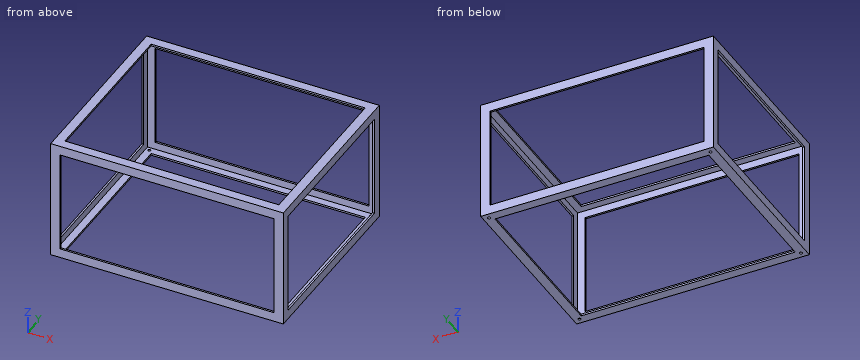
```python
from build123d import *

# Parameters (mm, degrees)
SKETCH1_W           = 250
SKETCH1_H           = 130
BOSS_EXTRUDE1_DEPTH = 200
SKETCH2_W           = 246
SKETCH2_H           = 126
CUT_EXTRUDE1_DEPTH  = 198
SKETCH3_W           = 230
SKETCH3_H           = 180
CUT_EXTRUDE2_DEPTH  = 3
SKETCH4_W           = 250
SKETCH4_H           = 2
BOSS_EXTRUDE2_DEPTH = 10
SKETCH5_W           = 110
SKETCH5_H           = 180
CUT_EXTRUDE3_DEPTH  = 3
SKETCH6_W           = 130
SKETCH6_H           = 2
BOSS_EXTRUDE3_DEPTH = 10
SKETCH7_W           = 230
SKETCH7_H           = 180
CUT_EXTRUDE4_DEPTH  = 3
SKETCH8_W           = 250
SKETCH8_H           = 2
BOSS_EXTRUDE4_DEPTH = 10
SKETCH9_W           = 110
SKETCH9_H           = 180
CUT_EXTRUDE5_DEPTH  = 3
SKETCH10_W          = 130
SKETCH10_H          = 2
BOSS_EXTRUDE5_DEPTH = 10
SKETCH11_W          = 230
SKETCH11_H          = 110
CUT_EXTRUDE7_DEPTH  = 3
SKETCH12_R          = 1.5
CUT_EXTRUDE8_DEPTH  = 3


with BuildPart() as part:
    # Sketch1 → Boss-Extrude1 (new body)
    with BuildSketch(Plane(origin=(0, 0, 0), x_dir=(1, 0, 0), z_dir=(0, 1, 0))):
        Rectangle(SKETCH1_W, SKETCH1_H)
    extrude(amount=BOSS_EXTRUDE1_DEPTH)

    # Sketch2 → Cut-Extrude1 (cut)
    with BuildSketch(Plane(origin=(0, 200, 0), x_dir=(1, 0, 0), z_dir=(0, 1, 0))):
        Rectangle(SKETCH2_W, SKETCH2_H)
    extrude(amount=-CUT_EXTRUDE1_DEPTH, mode=Mode.SUBTRACT)

    # Sketch3 → Cut-Extrude2 (cut)
    with BuildSketch(Plane.XY.offset(65)):
        with Locations((0, 100)):
            Rectangle(SKETCH3_W, SKETCH3_H)
    extrude(amount=-CUT_EXTRUDE2_DEPTH, mode=Mode.SUBTRACT)

    # Sketch4 → Boss-Extrude2 (add)
    with BuildSketch(Plane.XY.offset(65)):
        with Locations((0, 199)):
            Rectangle(SKETCH4_W, SKETCH4_H)
    extrude(amount=-BOSS_EXTRUDE2_DEPTH)

    # Sketch5 → Cut-Extrude3 (cut)
    with BuildSketch(Plane(origin=(125, 0, 0), x_dir=(0, 0, -1), z_dir=(1, 0, 0))):
        with Locations((0, 100)):
            Rectangle(SKETCH5_W, SKETCH5_H)
    extrude(amount=-CUT_EXTRUDE3_DEPTH, mode=Mode.SUBTRACT)

    # Sketch6 → Boss-Extrude3 (add)
    with BuildSketch(Plane(origin=(125, 0, 0), x_dir=(0, 0, -1), z_dir=(1, 0, 0))):
        with Locations((0, 199)):
            Rectangle(SKETCH6_W, SKETCH6_H)
    extrude(amount=-BOSS_EXTRUDE3_DEPTH)

    # Sketch7 → Cut-Extrude4 (cut)
    with BuildSketch(Plane(origin=(0, 0, -65), x_dir=(-1, 0, 0), z_dir=(0, 0, -1))):
        with Locations((0, 100)):
            Rectangle(SKETCH7_W, SKETCH7_H)
    extrude(amount=-CUT_EXTRUDE4_DEPTH, mode=Mode.SUBTRACT)

    # Sketch8 → Boss-Extrude4 (add)
    with BuildSketch(Plane(origin=(0, 0, -65), x_dir=(-1, 0, 0), z_dir=(0, 0, -1))):
        with Locations((0, 199)):
            Rectangle(SKETCH8_W, SKETCH8_H)
    extrude(amount=-BOSS_EXTRUDE4_DEPTH)

    # Sketch9 → Cut-Extrude5 (cut)
    with BuildSketch(Plane.ZY.offset(125)):
        with Locations((0, 100)):
            Rectangle(SKETCH9_W, SKETCH9_H)
    extrude(amount=-CUT_EXTRUDE5_DEPTH, mode=Mode.SUBTRACT)

    # Sketch10 → Boss-Extrude5 (add)
    with BuildSketch(Plane.ZY.offset(125)):
        with Locations((0, 199)):
            Rectangle(SKETCH10_W, SKETCH10_H)
    extrude(amount=-BOSS_EXTRUDE5_DEPTH)

    # Sketch11 → Cut-Extrude7 (cut)
    with BuildSketch(Plane.XZ):
        Rectangle(SKETCH11_W, SKETCH11_H)
    extrude(amount=-CUT_EXTRUDE7_DEPTH, mode=Mode.SUBTRACT)

    # Sketch12 → Cut-Extrude8 (cut)
    with BuildSketch(Plane(origin=(0, 0, -65), x_dir=(-1, 0, 0), z_dir=(0, 0, -1))):
        with Locations((-119, 194)):
            Circle(SKETCH12_R)
        with Locations((119, 194)):
            Circle(SKETCH12_R)
        with Locations((119, 6)):
            Circle(SKETCH12_R)
        with Locations((-119, 6)):
            Circle(SKETCH12_R)
    extrude(amount=-CUT_EXTRUDE8_DEPTH, mode=Mode.SUBTRACT)


solid = part.part
```
For this review, take the finished solid that the model builds, in its own axes (mm). Round coordinates to 2 decimals unless told otherwise and drop trailing zeros. Write each loop counter-clockwise with the first axis right and the second up, starting at its lowest first coordinate (ties: lowest second). Pieces come first, ordered by that corner, then holes. Notation, with made-up numbers: (-30.75, -34) -> (23.25, -34) arc R24 ccw to (23.25, -17) -> close; hole circle Ø2 at (4.25, -29). An arc over 180 degrees is marked (long way). One line per question, with ' | ' between items. Start each with the question number.
(1) Add section B-B, the plane x = -14.5. Write out the cut boundary in (y, z), plus the area to 3 significant figures.
(2) For line 1 along Y through (x, z) = (119, -64); line 2 along X through (y, z) = (194, -63.6); line 3 along X through (y, z) = (28.5, -57), list the stretches that pass through material, from the lowest coordinate up. Write a range as from..to.
(3) Add section A-A, the plane y = 112.5. Write out the cut boundary in (x, z).
Answer list:
1) outline: (0, -65) -> (10, -65) -> (10, -63) -> (2, -63) -> (2, -55) -> (0, -55) -> close; (0, 55) -> (2, 55) -> (2, 63) -> (10, 63) -> (10, 65) -> (0, 65) -> close; (190, -65) -> (200, -65) -> (200, -55) -> (198, -55) -> (198, -63) -> (190, -63) -> close; (190, 63) -> (198, 63) -> (198, 55) -> (200, 55) -> (200, 65) -> (190, 65) -> close | area: 144 mm²
2) line 1: 0..4.5, 7.5..192.5, 195.5..200 | line 2: -125..-120.5, -117.5..117.5, 120.5..125 | line 3: -125..-123, 123..125
3) outline: (-125, -65) -> (-115, -65) -> (-115, -63) -> (-123, -63) -> (-123, -55) -> (-125, -55) -> close; (-125, 55) -> (-123, 55) -> (-123, 63) -> (-115, 63) -> (-115, 65) -> (-125, 65) -> close; (115, -65) -> (125, -65) -> (125, -55) -> (123, -55) -> (123, -63) -> (115, -63) -> close; (115, 63) -> (123, 63) -> (123, 55) -> (125, 55) -> (125, 65) -> (115, 65) -> close
